Check sheet for the modelled part. Datum: model origin and axes. Units: mm. Give positions to 0.01 mm unless a question says otherwise; leave off trailing zeros. Write each loop counter-clockwise with the first axis right and the second up, starting at its lowest first coordinate (ties: lowest second). Pieces come first, ordered by that corner, then holes. Notation, with made-up numbers: M 10,-25.75 L 66,-25.75 A17 cw 66,-15.75 Z; hole C 17,89.25 d1. An arc over 180 degrees is marked long. Use CSV: the item, a comma, the result in double quotes. Start each with the question number.
1. Scan lines: line 1 (X direction, y = 1.8, z = 90) (3 decimals); line 2 (Z direction, x = 174.5, y = 0.6); line 3 (X direction, y = 0.25, z = 196). Record each from-to range of solid material in increasing order.
2. Depth check by flat-ended pin: P1, Ø1.6, axis at x = 84, y = 1, coming from the -Z side; P2, Ø1, axis at y = 0.5, z = 122.5, coming from the +X side; P3, Ø1, axis at y = 1.5, z = 131.5, coming from the +X side. Enter the tip coordinate at first touch or a pass-through.
3. Mould release check, pull along X, two halves, no side actions. Record for faces 1 (the face through (254.133, 1.61, 158.641)), 2 (the face through (208.9, 1.6, 211.5)), 3 (the face through (217, 3.175, 209)), 4 (the face through (272.107, 1.565, 89.723)): +X half, -X half, draft (parallel to the pull), parting line (faces both ways), or undercut.
4. Cross-section at B-B, the plane x = 222.5. Enter the section's corners in (y, z) (3 decimals).
5. Cross-section at A-A, the plane y = 2.5. Enter the section's corners in (x, z) (3 decimals).
6. Cross-section at C-C, the plane z = 112. Enter the section's corners in (x, y) (3 decimals), and give its area (3 significant figures).
from build123d import *

# Parameters (mm, degrees)
SKETCH1_R           = 2.125
BOSS_EXTRUDE1_DEPTH = 3.175
CUT_EXTRUDE1_DEPTH  = 396.992525971
BOSS_EXTRUDE2_DEPTH = 3.175
SKETCH4_R           = 2.125
CUT_EXTRUDE2_DEPTH  = 396.992525971


with BuildPart() as part:
    # Sketch1 → Boss-Extrude1 (new body)
    with BuildSketch(Plane(origin=(0, 0, 0), x_dir=(1, 0, 0), z_dir=(0, 1, 0))):
        Polygon((0, -280), (100, -280), (100, -209.601551084), (209.601551084, -100), (280, -100), (280, 0), (280, 100), (209.601551084, 100), (100, 209.601551084), (100, 280), (0, 280), (-100, 280), (-100, 209.601551084), (-209.601551084, 100), (-280, 100), (-280, 0), (-280, -100), (-209.601551084, -100), (-100, -209.601551084), (-100, -280), align=None)
        with Locations(Location((-47.5, -192, 0), (0, 0, 270))):
            Circle(SKETCH1_R, mode=Mode.SUBTRACT)
        with Locations(Location((-47.5, -217, 0), (0, 0, 270))):
            Circle(SKETCH1_R, mode=Mode.SUBTRACT)
        with Locations(Location((47.5, -217, 0), (0, 0, 270))):
            Circle(SKETCH1_R, mode=Mode.SUBTRACT)
        with Locations(Location((47.5, -192, 0), (0, 0, 270))):
            Circle(SKETCH1_R, mode=Mode.SUBTRACT)
        with Locations(Location((-192, 47.5, 0), (0, 0, 270))):
            Circle(SKETCH1_R, mode=Mode.SUBTRACT)
        with Locations(Location((-217, 47.5, 0), (0, 0, 270))):
            Circle(SKETCH1_R, mode=Mode.SUBTRACT)
        with Locations(Location((-192, -47.5, 0), (0, 0, 270))):
            Circle(SKETCH1_R, mode=Mode.SUBTRACT)
        with Locations(Location((-217, -47.5, 0), (0, 0, 270))):
            Circle(SKETCH1_R, mode=Mode.SUBTRACT)
        with Locations(Location((47.5, 192, 0), (0, 0, 270))):
            Circle(SKETCH1_R, mode=Mode.SUBTRACT)
        with Locations(Location((47.5, 217, 0), (0, 0, 270))):
            Circle(SKETCH1_R, mode=Mode.SUBTRACT)
        with Locations(Location((-47.5, 192, 0), (0, 0, 270))):
            Circle(SKETCH1_R, mode=Mode.SUBTRACT)
        with Locations(Location((-47.5, 217, 0), (0, 0, 270))):
            Circle(SKETCH1_R, mode=Mode.SUBTRACT)
        with Locations(Location((192, -47.5, 0), (0, 0, 270))):
            Circle(SKETCH1_R, mode=Mode.SUBTRACT)
        with Locations(Location((217, -47.5, 0), (0, 0, 270))):
            Circle(SKETCH1_R, mode=Mode.SUBTRACT)
        with Locations(Location((192, 47.5, 0), (0, 0, 270))):
            Circle(SKETCH1_R, mode=Mode.SUBTRACT)
        with Locations(Location((217, 47.5, 0), (0, 0, 270))):
            Circle(SKETCH1_R, mode=Mode.SUBTRACT)
        with Locations(Location((-90, -270, 0), (0, 0, 270))):
            Circle(SKETCH1_R, mode=Mode.SUBTRACT)
        with Locations(Location((-30, -270, 0), (0, 0, 270))):
            Circle(SKETCH1_R, mode=Mode.SUBTRACT)
        with Locations(Location((30, -270, 0), (0, 0, 270))):
            Circle(SKETCH1_R, mode=Mode.SUBTRACT)
        with Locations(Location((90, -270, 0), (0, 0, 270))):
            Circle(SKETCH1_R, mode=Mode.SUBTRACT)
        with Locations(Location((-270, 90, 0), (0, 0, 270))):
            Circle(SKETCH1_R, mode=Mode.SUBTRACT)
        with Locations(Location((-270, 30, 0), (0, 0, 270))):
            Circle(SKETCH1_R, mode=Mode.SUBTRACT)
        with Locations(Location((-270, -30, 0), (0, 0, 270))):
            Circle(SKETCH1_R, mode=Mode.SUBTRACT)
        with Locations(Location((-270, -90, 0), (0, 0, 270))):
            Circle(SKETCH1_R, mode=Mode.SUBTRACT)
        with Locations(Location((90, 270, 0), (0, 0, 270))):
            Circle(SKETCH1_R, mode=Mode.SUBTRACT)
        with Locations(Location((30, 270, 0), (0, 0, 270))):
            Circle(SKETCH1_R, mode=Mode.SUBTRACT)
        with Locations(Location((-30, 270, 0), (0, 0, 270))):
            Circle(SKETCH1_R, mode=Mode.SUBTRACT)
        with Locations(Location((-90, 270, 0), (0, 0, 270))):
            Circle(SKETCH1_R, mode=Mode.SUBTRACT)
        with Locations(Location((270, -90, 0), (0, 0, 270))):
            Circle(SKETCH1_R, mode=Mode.SUBTRACT)
        with Locations(Location((270, -30, 0), (0, 0, 270))):
            Circle(SKETCH1_R, mode=Mode.SUBTRACT)
        with Locations(Location((270, 30, 0), (0, 0, 270))):
            Circle(SKETCH1_R, mode=Mode.SUBTRACT)
        with Locations(Location((270, 90, 0), (0, 0, 270))):
            Circle(SKETCH1_R, mode=Mode.SUBTRACT)
        with Locations(Location((-90, -250, 0), (0, 0, 270))):
            Circle(SKETCH1_R, mode=Mode.SUBTRACT)
        with Locations(Location((-90, -180, 0), (0, 0, 270))):
            Circle(SKETCH1_R, mode=Mode.SUBTRACT)
        with Locations(Location((-90, -110, 0), (0, 0, 270))):
            Circle(SKETCH1_R, mode=Mode.SUBTRACT)
        with Locations(Location((-90, -40, 0), (0, 0, 270))):
            Circle(SKETCH1_R, mode=Mode.SUBTRACT)
        with Locations(Location((-90, 30, 0), (0, 0, 270))):
            Circle(SKETCH1_R, mode=Mode.SUBTRACT)
        with Locations(Location((-90, 50, 0), (0, 0, 270))):
            Circle(SKETCH1_R, mode=Mode.SUBTRACT)
        with Locations(Location((-90, 150, 0), (0, 0, 270))):
            Circle(SKETCH1_R, mode=Mode.SUBTRACT)
        with Locations(Location((-90, 250, 0), (0, 0, 270))):
            Circle(SKETCH1_R, mode=Mode.SUBTRACT)
        with Locations(Location((90, -250, 0), (0, 0, 270))):
            Circle(SKETCH1_R, mode=Mode.SUBTRACT)
        with Locations(Location((90, -180, 0), (0, 0, 270))):
            Circle(SKETCH1_R, mode=Mode.SUBTRACT)
        with Locations(Location((90, -110, 0), (0, 0, 270))):
            Circle(SKETCH1_R, mode=Mode.SUBTRACT)
        with Locations(Location((90, -40, 0), (0, 0, 270))):
            Circle(SKETCH1_R, mode=Mode.SUBTRACT)
        with Locations(Location((90, 30, 0), (0, 0, 270))):
            Circle(SKETCH1_R, mode=Mode.SUBTRACT)
        with Locations(Location((90, 50, 0), (0, 0, 270))):
            Circle(SKETCH1_R, mode=Mode.SUBTRACT)
        with Locations(Location((90, 150, 0), (0, 0, 270))):
            Circle(SKETCH1_R, mode=Mode.SUBTRACT)
        with Locations(Location((90, 250, 0), (0, 0, 270))):
            Circle(SKETCH1_R, mode=Mode.SUBTRACT)
        with Locations(Location((-250, -90, 0), (0, 0, 270))):
            Circle(SKETCH1_R, mode=Mode.SUBTRACT)
        with Locations(Location((-180, -90, 0), (0, 0, 270))):
            Circle(SKETCH1_R, mode=Mode.SUBTRACT)
        with Locations(Location((-110, -90, 0), (0, 0, 270))):
            Circle(SKETCH1_R, mode=Mode.SUBTRACT)
        with Locations(Location((-110, 90, 0), (0, 0, 270))):
            Circle(SKETCH1_R, mode=Mode.SUBTRACT)
        with Locations(Location((-180, 90, 0), (0, 0, 270))):
            Circle(SKETCH1_R, mode=Mode.SUBTRACT)
        with Locations(Location((-250, 90, 0), (0, 0, 270))):
            Circle(SKETCH1_R, mode=Mode.SUBTRACT)
        with Locations(Location((110, -90, 0), (0, 0, 270))):
            Circle(SKETCH1_R, mode=Mode.SUBTRACT)
        with Locations(Location((180, -90, 0), (0, 0, 270))):
            Circle(SKETCH1_R, mode=Mode.SUBTRACT)
        with Locations(Location((250, -90, 0), (0, 0, 270))):
            Circle(SKETCH1_R, mode=Mode.SUBTRACT)
        with Locations(Location((110, 90, 0), (0, 0, 270))):
            Circle(SKETCH1_R, mode=Mode.SUBTRACT)
        with Locations(Location((180, 90, 0), (0, 0, 270))):
            Circle(SKETCH1_R, mode=Mode.SUBTRACT)
        with Locations(Location((250, 90, 0), (0, 0, 270))):
            Circle(SKETCH1_R, mode=Mode.SUBTRACT)
    extrude(amount=BOSS_EXTRUDE1_DEPTH)

    # Sketch2 → Cut-Extrude1 (cut, through all)
    with BuildSketch(Plane(origin=(0, 3.175, 0), x_dir=(1, 0, 0), z_dir=(0, 1, 0))):
        Polygon((80, -260), (100, -260), (100, -209.601551084), (209.601551084, -100), (260, -100), (260, -80), (280, -80), (280, 100), (209.601551084, 100), (100, 209.601551084), (100, 280), (-100, 280), (-100, 209.601551084), (-209.601551084, 100), (-280, 100), (-280, -100), (-209.601551084, -100), (-100, -209.601551084), (-100, -280), (80, -280), align=None)
    extrude(amount=-CUT_EXTRUDE1_DEPTH, mode=Mode.SUBTRACT)


with BuildPart() as cut_extrude1_piece_1:
    # of the separate pieces the step leaves, piece 1, a body of its own (cut_extrude1_pieces)
    add(part.part.solids().sort_by_distance((100, 0, 280))[0])



with BuildPart() as cut_extrude1_piece_2:
    # of the separate pieces the step leaves, piece 2, a body of its own (cut_extrude1_pieces)
    add(part.part.solids().sort_by_distance((260, 3.175, 100))[0])


with BuildPart() as cut_extrude1_piece_1_1:
    add(cut_extrude1_piece_1.part)

    add(cut_extrude1_piece_2.part)  # Boss-Extrude2 merges Cut-Extrude1 piece 2
    # Sketch3 → Boss-Extrude2 (add)
    with BuildSketch(Plane(origin=(0, 3.175, 0), x_dir=(1, 0, 0), z_dir=(0, 1, 0))):
        with BuildLine():
            Line((260, -90), (267.875, -90))
            ThreePointArc((267.875, -90), (270, -92.125), (272.125, -90))
            Line((272.125, -90), (280, -90))
            ThreePointArc((280, -90), (224.350288425, -224.350288425), (90, -280))
            Line((90, -280), (90, -272.125))
            ThreePointArc((90, -272.125), (92.125, -270), (90, -267.875))
            Line((90, -267.875), (90, -260))
            ThreePointArc((90, -260), (210.208152802, -210.208152802), (260, -90))
        make_face()
    extrude(amount=-BOSS_EXTRUDE2_DEPTH)

    # Sketch4 → Cut-Extrude2 (cut, through all)
    with BuildSketch(Plane(origin=(0, 3.175, 0), x_dir=(1, 0, 0), z_dir=(0, 1, 0))):
        with Locations(Location((217.279220614, -217.279220614, 0), (0, 0, 270))):
            Circle(SKETCH4_R)
        with Locations(Location((256.207454383, -159.101968912, 0), (0, 0, 270))):
            Circle(SKETCH4_R)
        with Locations(Location((159.101968912, -256.207454383, 0), (0, 0, 90))):
            Circle(SKETCH4_R)
        with BuildLine():
            Line((100, -280), (90, -280))
            ThreePointArc((90, -280), (95.001733404, -279.934153493), (100, -279.73665961))
            Line((100, -279.73665961), (100, -280))
        make_face()
        with BuildLine():
            Line((279.73665961, -100), (284.415704741, -100))
            Line((284.415704741, -100), (280, -90))
            ThreePointArc((280, -90), (279.934153493, -95.001733404), (279.73665961, -100))
        make_face()
    extrude(amount=-CUT_EXTRUDE2_DEPTH, mode=Mode.SUBTRACT)


solid = cut_extrude1_piece_1_1.part
Worked answers:
1,line 1,"x = 260 to 267.875, 272.125 to 280"
1,line 2,"z = 237.51 to 260.18"
1,line 3,"x = 222.91 to 247.68"
2,P1,"stops at z = 260"
2,P2,"stops at x = 277.29"
2,P3,"stops at x = 275.52"
3,face 1,"undercut"
3,face 2,"-X half"
3,face 3,"draft"
3,face 4,"undercut"
4,outline,"M 0,196.507 L 3.175,196.507 L 3.175,226.175 L 0,226.175 Z"
5,outline,"M 80,260 L 90,260 A170 cw 260,90 L 260,80 L 280,80 L 280,90 A190 ccw 279.737,100 A190 ccw 100,279.737 A190 ccw 90,280 L 80,280 Z; hole C 90,270 d4.25; hole C 159.102,256.207 d4.25; hole C 217.279,217.279 d4.25; hole C 256.207,159.102 d4.25; hole C 270,90 d4.25"
6,outline,"M 258.57,0 L 278.722,0 L 278.722,3.175 L 258.57,3.175 Z"
6,area,"64.0 mm^2"
